Can you work these out from the drawing? Everything is in mm from the part's minimum corner. A direction names the side the tool comes from. Coordinates: 2 decimals unless noted, no trailing zeros. Loops run counter-clockwise (first coordinate to the right, second up) from the corner with the lowest first, then second, coordinate; pieces in that order, holes last. Notation, with made-up numbers: (-1.5, 23.25) - (6.5, 23.25) arc R16 cw to (6.5, 30.25) - close; hole circle Ø4 at (10, 70). An arc over 180 degrees is marked (long way). Put each result on its own line as item: value. Start each with the question number.
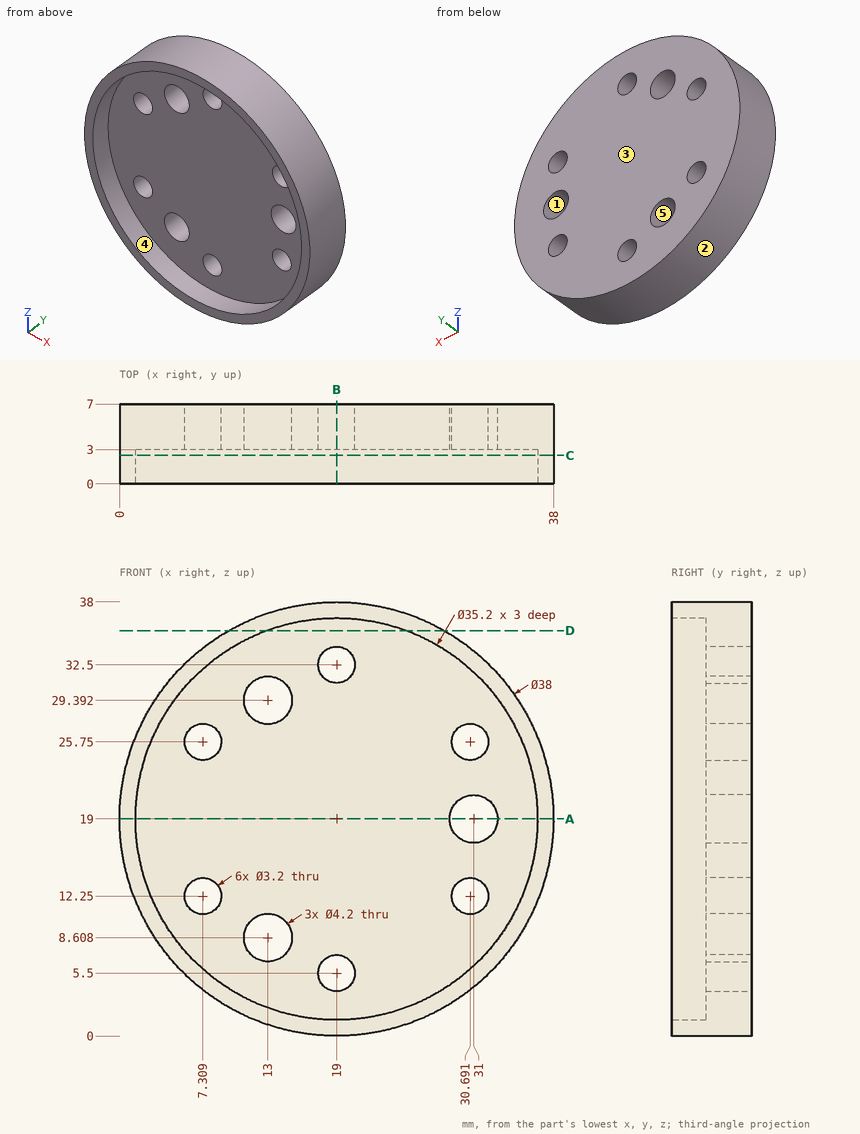
Q1. I want a section at C-C on y = 2.5. List the corners of the cut face in (x, z) for me, and give its area (3 significant figures).
Q2. We'd pull the mould along Z, two halves only. Please class the marked faces 1, 2 and 3: released by +Z, released by -Z, zero draft, split by the parting line, or undercut.
Q3. Will these pins go through, and if not, where does the flat tip stop? pin 1 (3 mm diameter, centred on x = 17.5, y = 1.5, fed in from -Z); pin 2 (2 mm diameter, centred on y = 1.5, z = 10.5, fed in from -X); pin 3 (4 mm diameter, centred on y = 3, z = 31.5, fed in from -X) (1 decimal); pin 4 (3 mm diameter, centred on x = 28.5, y = 2, fed in from +Z).
Q4. I want a section at B-B on x = 19. List the corners of the cut face in (y, z) for me.
Q5. Please list where these lines run through material, in increasing order: line 1 along X through (y, z) = (5.5, 12.25); line 2 along Y through (x, z) = (4, 28); line 3 along Z through (x, y) = (6, 5.5) (1 decimal). Write a range as [from, to].
Q6. I want a section at D-D on z = 35.5. List the corners of the cut face in (x, y) for me (1 decimal).
Q7. On a 3-axis mill with a long thin cutter (end or side, diameter ignored), from which of +Z, -Z, +X, -X, +Y, -Y can I reach the whole of each face in a straight line? I mean the marked faces 4 and 5. Say none if no direction works.
Q8. I want a section at A-A on z = 19. List the corners of the cut face in (x, y) for me, and give its area (3 significant figures).
Calculated:
1. outline: circle Ø38 at (19, 19); hole circle Ø35.2 at (19, 19)
1. area: 161 mm2
2. face 1: undercut
2. face 2: split by the parting line
2. face 3: zero draft
3. pin 1: z = 0
3. pin 2: x = 1.54
3. pin 3: x = 3.2
3. pin 4: z = 36.23
4. outline: (0, 0) - (7, 0) - (7, 3.9) - (3, 3.9) - (3, 1.4) - (0, 1.4) - close; (0, 36.6) - (3, 36.6) - (3, 34.1) - (7, 34.1) - (7, 38) - (0, 38) - close; (3, 7.1) - (7, 7.1) - (7, 30.9) - (3, 30.9) - close
5. line 1: [1.24, 5.71], [8.91, 29.09], [32.29, 36.76]
5. line 2: [3, 7]
5. line 3: [5.1, 11.3], [13.2, 24.8], [26.7, 32.9]
6. outline: (9.6, 0) - (12.9, 0) - (12.9, 3) - (25.1, 3) - (25.1, 0) - (28.4, 0) - (28.4, 7) - (9.6, 7) - close
7. face 4: -Y
7. face 5: +Y, -Y
8. outline: (0, 0) - (1.4, 0) - (1.4, 3) - (28.9, 3) - (28.9, 7) - (0, 7) - close; (33.1, 3) - (36.6, 3) - (36.6, 0) - (38, 0) - (38, 7) - (33.1, 7) - close
8. area: 144 mm2
